Read the model definition and answer for the solid it produces. Units are mm, in the model's axes. Face numbers are marked on the shaded views. A direction names the side the tool comes from. Give positions to 0.01 mm unless a question says otherwise; leave off trailing zeros. Write each loop counter-clockwise with the first axis right and the second up, starting at its lowest first coordinate (ties: lowest second). Pieces come first, ordered by that corner, then holes. Notation, with made-up numbers: (72.25, 26.25) -> (129.25, 26.25) arc R19 cw to (129.25, 33.25) -> close; hole circle Ø2 at (-34.75, 64). An arc over 180 degrees is marked (long way). Answer as CSV lines item,"result". Start each with the question number.
1. A tool of negligible diameter and unlimited length cuts with its end or side. For the marked faces 4, 5 and 6, from which of +Z, -Z, +X, -X, +Y, -Y can it reach the whole face along a straight path? Write none if from no direction.
2. The part is cut by section C-C, the plane z = 0. Give the number of separate pieces and of enclosed holes in the cut face, and give its area (3 significant figures).
3. The part is cut by section D-D, the plane x = 38.1. Determine the outline of the cut face in (y, z), and give its area (3 significant figures).
4. Find the intervals of material crossed by line 1 (X direction, y = -16, z = 0); line 2 (X direction, y = -24, z = 0) (3 decimals); line 3 (Z direction, x = 0, y = -14), in increasing order.
5. For a pull along Z with two mould halves and no side action, classify the marked faces 1, 2 and 3 as pulls with the +Z half, pulls with the -Z half, needs draft (parallel to the pull), parting line crosses it, or undercut.
6. The part is cut by section B-B, the plane y = -31. Determine the outline of the cut face in (x, z), and give its area (3 significant figures).
7. Given pin 1 (20.5 mm diameter, centred on x = 0, z = 0, fed in from -Y); pin 2 (6 mm diameter, centred on y = -20, z = -35, fed in from -X); pin 3 (18.5 mm diameter, centred on x = 38.1, z = 0, fed in from -Y); pin 4 (8.5 mm diameter, centred on x = -38.1, z = 0, fed in from -Y), each flat-ended and moving along its own axis, determine where each tip first touches the part or whether it passes through.
8. The part is cut by section A-A, the plane x = 0. Determine the outline of the cut face in (y, z) (3 decimals), and give its area (3 significant figures).
from build123d import *

# Parameters (mm, degrees)
F_3_8_NPT_TAPPED_HOLE1_AT_2_COUNT = 2
F_3_8_NPT_TAPPED_HOLE1_AT_2_PITCH = 76.2


with BuildPart() as part:
    # Sketch1 → Revolve1 (revolve)
    with BuildSketch(Plane.XY):
        Polygon((0, 0), (-76.2, 0), (-76.2, -38.1), (-60.96, -38.1), (-60.96, -25.4), (-28.575, -25.4), (-28.575, -20.32), (-22.225, -20.32), (0, -15.85722), align=None)
    revolve(axis=Axis((0, 0, 0), (0, -1, 0)))

    # Sketch3 → 1/2 NPT Tapped Hole1 (revolve, cut)
    with BuildSketch(Plane(origin=(0, 0, 0), x_dir=(0, 0, 1), z_dir=(1, 0, 0))):
        Polygon((0, 0), (0, 38.1), (8.9281, 38.1), (8.9281, 13.462), (10.261665792, 13.462), (10.6647361, 0), align=None)
    revolve(axis=Axis((0, 6.35, 0), (0, -1, 0)), mode=Mode.SUBTRACT)

    # Sketch5 → 3/8 NPT Tapped Hole1 (revolve, cut)
    with BuildSketch(Plane(origin=(-38.1, 0, 0), x_dir=(0, 0, 1), z_dir=(1, 0, 0))):
        Polygon((0, 0), (0, 38.1), (7.1374, 38.1), (7.1374, 10.414), (8.263205494, 10.414), (8.5750146, 0), align=None)
    f_3_8_npt_tapped_hole1 = revolve(axis=Axis((-38.1, 6.35, 0), (0, -1, 0)), mode=Mode.SUBTRACT)

    # 3/8 NPT Tapped Hole1 at 2: 3/8 NPT Tapped Hole1 ×2
    with Locations(*[(i * F_3_8_NPT_TAPPED_HOLE1_AT_2_PITCH, 0, 0) for i in range(1, F_3_8_NPT_TAPPED_HOLE1_AT_2_COUNT)]):
        add(f_3_8_npt_tapped_hole1, mode=Mode.SUBTRACT)


solid = part.part
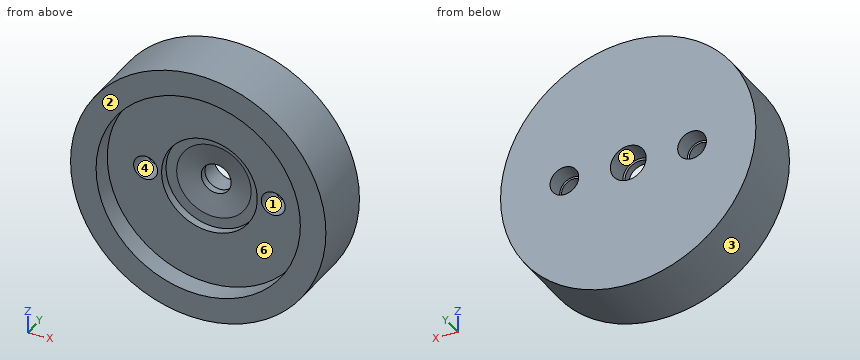
Results found:
1,face 4,"+Y, -Y"
1,face 5,"+Y"
1,face 6,"-Y"
2,separate pieces,"4"
2,enclosed holes,"0"
2,area,"2,750 mm²"
3,outline,"(-38.1, -65.99) -> (0, -65.99) -> (0, -8.58) -> (-10.41, -8.26) -> (-10.41, -7.14) -> (-25.4, -7.14) -> (-25.4, -47.59) -> (-38.1, -47.59) -> close; (-38.1, 47.59) -> (-25.4, 47.59) -> (-25.4, 7.14) -> (-10.41, 7.14) -> (-10.41, 8.26) -> (0, 8.58) -> (0, 65.99) -> (-38.1, 65.99) -> close"
3,area,"3,430 mm²"
4,line 1,"x = -76.2 to -45.24, -30.96 to -8.93, 8.93 to 30.96, 45.24 to 76.2"
4,line 2,"x = -76.2 to -45.237, -30.963 to -28.575, 28.575 to 30.963, 45.237 to 76.2"
4,line 3,"z = -76.2 to -8.93, 8.93 to 76.2"
5,face 1,"undercut"
5,face 2,"needs draft"
5,face 3,"parting line crosses it"
6,outline,"circle Ø152.4 at (0, 0); hole circle Ø121.92 at (0, 0)"
6,area,"6,570 mm²"
7,pin 1,"stops at y = -17.92"
7,pin 2,"stops at x = -69.16"
7,pin 3,"stops at y = -25.4"
7,pin 4,"passes through"
8,outline,"(-38.1, -76.2) -> (0, -76.2) -> (0, -10.665) -> (-13.462, -10.262) -> (-13.462, -8.928) -> (-17.65, -8.928) -> (-20.32, -22.225) -> (-20.32, -28.575) -> (-25.4, -28.575) -> (-25.4, -60.96) -> (-38.1, -60.96) -> close; (-38.1, 60.96) -> (-25.4, 60.96) -> (-25.4, 28.575) -> (-20.32, 28.575) -> (-20.32, 22.225) -> (-17.65, 8.928) -> (-13.462, 8.928) -> (-13.462, 10.262) -> (0, 10.665) -> (0, 76.2) -> (-38.1, 76.2) -> close"
8,area,"3,530 mm²"
